Build history of the part. All positions in model axes, mm. Face numbers are marked on the shaded views. A direction names the side the tool comes from. Coordinates: 2 decimals unless noted, no trailing zeros. Loops run counter-clockwise (first coordinate to the right, second up) from the corner with the lowest first, then second, coordinate; pieces in that order, holes last.
(1) Tool access for the marked faces 1, 2 and 3: list every direction of +Z, -Z, +X, -X, +Y, -Y with a clear straight run to the whole face (end or side of a thin tool).
(2) Slice it at B-B (x = -26). Give the cut face in (y, z), and give its area (3 significant figures).
(3) Wall check: L1, parallel to Y at x = 0, z = -0.75 (1 decimal); L2, parallel to X at y = 0, z = -2.5 (1 decimal); L3, parallel to Z at x = 19.5, y = 5.5. Give the ranges that are in metal, low to high.
(4) Flat gauge pins, fed straight in: P1, Ø1.8, axis at x = -0.5, z = -1, coming from the -Y side (3 decimals); P2, Ø2, axis at y = 5.5, z = 3.5, coming from the -X side; P3, Ø1, axis at x = 14, z = 0, coming from the -Y side. Where does each tip first touch, or does it go through?
(5) Slice it at C-C (y = -6). Give the cut face in (x, z).
from build123d import *

# Parameters (mm, degrees)
BOSS_EXTRUDE1_DEPTH = 6.35
BOSS_EXTRUDE2_START = -11.1125
SKETCH2_R           = 3.175
BOSS_EXTRUDE2_DEPTH = 11.1125


with BuildPart() as part:
    # Sketch1 → Boss-Extrude1 (new body)
    with BuildSketch(Plane.XY):
        with BuildLine():
            Line((15.026842649, 0), (30.48, 0))
            ThreePointArc((30.48, 0), (31.684827789, 0.868390737), (31.242, 2.286))
            ThreePointArc((31.242, 2.286), (16.465979776, 10.027939329), (0, 12.7))
            ThreePointArc((0, 12.7), (-8.197814749, 9.699785221), (-12.522368874, 2.116666667))
            ThreePointArc((-12.522368874, 2.116666667), (-13.387279699, 0.600042956), (-15.026842649, 0))
            Line((-15.026842649, 0), (-30.48, 0))
            ThreePointArc((-30.48, 0), (-31.684827789, -0.868390737), (-31.242, -2.286))
            ThreePointArc((-31.242, -2.286), (-16.465979776, -10.027939329), (0, -12.7))
            ThreePointArc((0, -12.7), (8.197814749, -9.699785221), (12.522368874, -2.116666667))
            ThreePointArc((12.522368874, -2.116666667), (13.387279699, -0.600042956), (15.026842649, 0))
        make_face()
        with BuildLine():
            Line((-1.107160332, 0.9525), (1.107160332, 0.9525))
            ThreePointArc((1.107160332, 0.9525), (0, -1.4605), (-1.107160332, 0.9525))
        make_face(mode=Mode.SUBTRACT)
    extrude(amount=BOSS_EXTRUDE1_DEPTH)

    # Sketch2 → Boss-Extrude2 (add)
    with BuildSketch(Plane.XY.offset(6.35).offset(BOSS_EXTRUDE2_START)):
        Circle(SKETCH2_R)
        with BuildLine():
            Line((-1.107160332, 0.9525), (1.107160332, 0.9525))
            ThreePointArc((1.107160332, 0.9525), (0, -1.4605), (-1.107160332, 0.9525))
        make_face(mode=Mode.SUBTRACT)
    extrude(amount=BOSS_EXTRUDE2_DEPTH)


solid = part.part
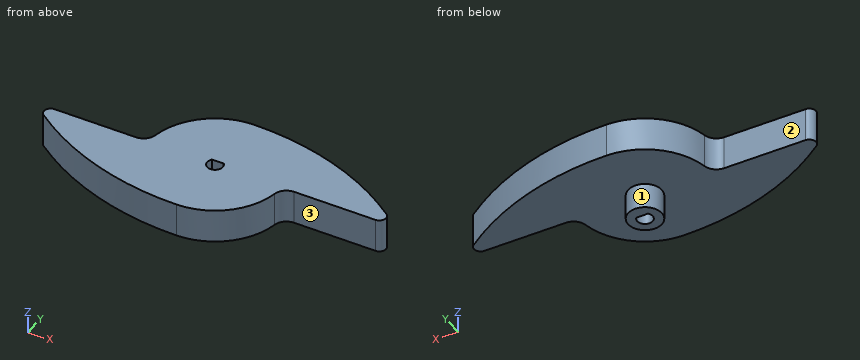
Response values:
1. face 1: -Z
1. face 2: +Z, -Z, -X, +Y
1. face 3: +Z, -Z, +X, -Y
2. outline: (-5.74, 0) - (0, 0) - (0, 6.35) - (-5.74, 6.35) - close
2. area: 36.5 mm2
3. L1: y = -3.2 to -1.5, 1 to 3.2
3. L2: x = -3.2 to -1.5, 1.5 to 3.2
3. L3: z = 0 to 6.35
4. P1: stops at y = -3.175
4. P2: stops at x = -11.88
4. P3: stops at y = -0.51
5. outline: (-25.55, 0) - (11.19, 0) - (11.19, 6.35) - (-25.55, 6.35) - close
